The figure shows three views and two pictorial views of one solid part (mm, origin at its lowest corner). Answer the questions. A direction names the side the tool comes from. Coordinates: 2 decimals unless noted, no trailing zeros. Loops run counter-clockwise (first coordinate to the right, second up) from the corner with the lowest first, then second, coordinate; pieces in that order, holes last. Notation, with made-up numbers: (52, 66.25) - (57, 66.25) arc R21 cw to (57, 70.25) - close; hole circle Ø10 at (-27, -33). An arc over 180 degrees is marked (long way). Write each question's results on one line, items separated by ' | '. Start each with the question number.
Item 1: Section C-C, the plane z = 4.75 is taken. Write down the section's boundary in (x, y) (3 decimals).
Item 2: A tool of negligible diameter and unlimited length cuts with its end or side. For the marked faces 4, 5 and 6, from which of +Z, -Z, +X, -X, +Y, -Y can it reach the whole face along a straight path? Write none if from no direction.
Item 3: For a pull along X with two mould halves and no side action, classify the marked faces 1, 2 and 3 as +X half, -X half, draft (parallel to the pull), parting line (faces both ways), or undercut.
Item 4: Section D-D, the plane y = 8.25 is taken. Write down the section's boundary in (x, z).
Item 5: Section A-A, the plane x = 18.75 is taken. Write down the section's boundary in (y, z).
Item 6: Each of these flat-tipped pins is pushed along its axis until it touches: pin 1 Ø3 at (x, y) = (16.845, 2.4) entering from -Z; pin 2 Ø2.5 at (x, z) = (11, 3.5) entering from +Y; pin 3 Ø1 at (x, z) = (20, 8.5) entering from +Y. Where does it stop, or does it pass through?
Item 7: Consider probe 1 along Z at (x, y) = (15.75, 3.5); probe 2 along X at (y, z) = (9, 7.5); probe 3 along X at (y, z) = (2.5, 19.5). Determine where each line is inside the solid, lowest interval first. Write a range as [from, to].
Item 8: Section B-B, the plane y = 2.4 is taken. Write down the section's boundary in (x, z).
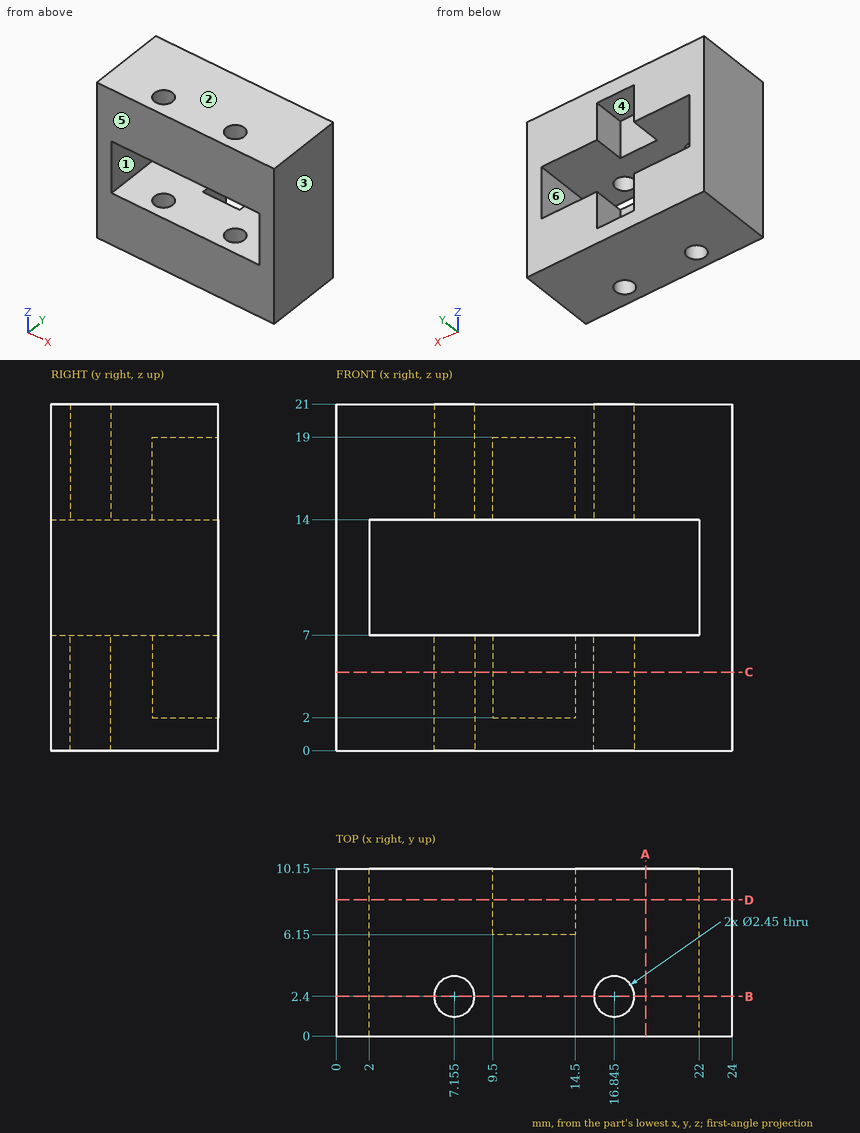
Answer key:
1) outline: (0, 0) - (24, 0) - (24, 10.15) - (14.5, 10.15) - (14.5, 6.15) - (9.5, 6.15) - (9.5, 10.15) - (0, 10.15) - close; hole circle Ø2.45 at (7.155, 2.4); hole circle Ø2.45 at (16.845, 2.4)
2) face 4: +Y | face 5: +Z, -Z, +X, -X, -Y | face 6: +Y, -Y
3) face 1: undercut | face 2: draft | face 3: +X half
4) outline: (0, 0) - (24, 0) - (24, 21) - (0, 21) - close; hole (2, 7) - (9.5, 7) - (9.5, 2) - (14.5, 2) - (14.5, 7) - (22, 7) - (22, 14) - (14.5, 14) - (14.5, 19) - (9.5, 19) - (9.5, 14) - (2, 14) - close
5) outline: (0, 0) - (10.15, 0) - (10.15, 7) - (0, 7) - close; (0, 14) - (10.15, 14) - (10.15, 21) - (0, 21) - close
6) pin 1: stops at z = 0 | pin 2: stops at y = 6.15 | pin 3: passes through
7) probe 1: z = [0, 7], [14, 21] | probe 2: x = [0, 2], [22, 24] | probe 3: x = [0, 5.93], [8.38, 15.62], [18.07, 24]
8) outline: (0, 0) - (5.93, 0) - (5.93, 7) - (2, 7) - (2, 14) - (5.93, 14) - (5.93, 21) - (0, 21) - close; (8.38, 0) - (15.62, 0) - (15.62, 7) - (8.38, 7) - close; (8.38, 14) - (15.62, 14) - (15.62, 21) - (8.38, 21) - close; (18.07, 0) - (24, 0) - (24, 21) - (18.07, 21) - (18.07, 14) - (22, 14) - (22, 7) - (18.07, 7) - close
